Can you work these out from the model? Positions are in its coordinate system, mm. Face numbers are marked on the shaded views. Coordinates: 2 decimals unless noted, no trailing zeros. Order: outer loops, then holes, each group sorted by start corner. A loop starts at its lowest first (then second) coordinate and runs counter-clockwise, first axis right, second up. Notation, with made-up numbers: (72.25, 49) -> (88.25, 49) arc R17 ccw to (88.25, 66) -> close; hole circle Ø4 at (-8, 41). An arc over 180 degrees is marked (long way). Write item = value, one per line.
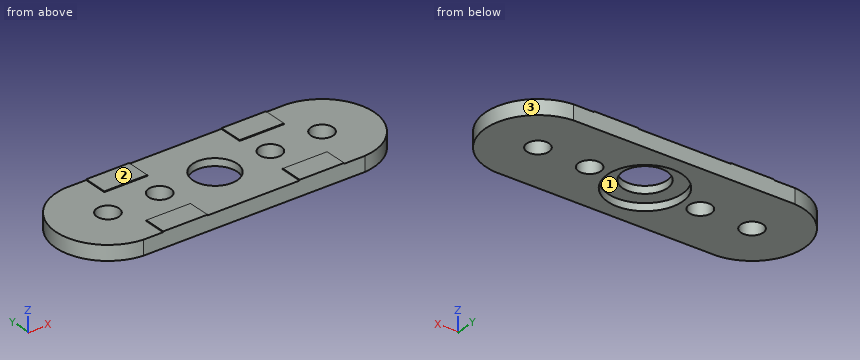
```python
from build123d import *

# Parameters (mm, degrees)
SKETCH1_R           = 3
SKETCH1_R_2         = 1.5
BOSS_EXTRUDE1_DEPTH = 2
SKETCH2_W           = 6.020555891
SKETCH2_H           = 3.042269969
SKETCH2_H_2         = 3.263297615
SKETCH2_W_2         = 6
SKETCH2_W_3         = 5.83801195
BOSS_EXTRUDE2_DEPTH = 0.1
SKETCH3_R           = 5
CUT_EXTRUDE1_DEPTH  = 1


with BuildPart() as part:
    # Sketch1 → Boss-Extrude1 (new body)
    with BuildSketch(Plane.XY):
        with BuildLine():
            Line((-15, -7), (15, -7))
            ThreePointArc((15, -7), (21.517834424, 0), (15, 7))
            Line((15, 7), (-15, 7))
            ThreePointArc((-15, 7), (-21.517834424, 0), (-15, -7))
        make_face()
        Circle(SKETCH1_R, mode=Mode.SUBTRACT)
        with Locations((-14.5, 0)):
            Circle(SKETCH1_R_2, mode=Mode.SUBTRACT)
        with Locations((14.5, 0)):
            Circle(SKETCH1_R_2, mode=Mode.SUBTRACT)
        with Locations((-7.5, 0)):
            Circle(SKETCH1_R_2, mode=Mode.SUBTRACT)
        with Locations((7.5, 0)):
            Circle(SKETCH1_R_2, mode=Mode.SUBTRACT)
    extrude(amount=BOSS_EXTRUDE1_DEPTH)

    # Sketch2 → Boss-Extrude2 (add)
    with BuildSketch(Plane.XY.offset(2)):
        with Locations((9.181574615, -5.478865016)):
            Rectangle(SKETCH2_W, SKETCH2_H)
        with Locations((9.181574615, 5.368351193)):
            Rectangle(SKETCH2_W, SKETCH2_H_2)
        with Locations((-9.322339138, -5.478865016)):
            Rectangle(SKETCH2_W_2, SKETCH2_H)
        with Locations((-9.241345113, 5.368351193)):
            Rectangle(SKETCH2_W_3, SKETCH2_H_2)
    extrude(amount=BOSS_EXTRUDE2_DEPTH)

    # Sketch3 → Cut-Extrude1 (cut)
    with BuildSketch(Plane(origin=(0, 0, 0), x_dir=(-1, 0, 0), z_dir=(0, 0, -1))):
        Circle(SKETCH3_R)
    extrude(amount=-CUT_EXTRUDE1_DEPTH, mode=Mode.SUBTRACT)


solid = part.part
```
Item 1: I want a section at C-C, the plane z = 1.6. Please give me the cut outline in (x, y).
A:
outline = (-15, -7) -> (15, -7) arc R7.02 ccw to (15, 7) -> (-15, 7) arc R7.02 ccw to start; hole circle Ø3 at (-14.5, 0); hole circle Ø3 at (-7.5, 0); hole circle Ø6 at (0, 0); hole circle Ø3 at (7.5, 0); hole circle Ø3 at (14.5, 0)
Item 2: I want a section at B-B, the plane y = 0. Please give me the cut outline in (x, z), plus the area to 3 significant figures.
A:
outline = (-21.52, 0) -> (-16, 0) -> (-16, 2) -> (-21.52, 2) -> close; (-13, 0) -> (-9, 0) -> (-9, 2) -> (-13, 2) -> close; (-6, 0) -> (-5, 0) -> (-5, 1) -> (-3, 1) -> (-3, 2) -> (-6, 2) -> close; (3, 1) -> (5, 1) -> (5, 0) -> (6, 0) -> (6, 2) -> (3, 2) -> close; (9, 0) -> (13, 0) -> (13, 2) -> (9, 2) -> close; (16, 0) -> (21.52, 0) -> (21.52, 2) -> (16, 2) -> close
area = 46.1 mm2
Item 3: I want a section at D-D, the plane y = 2. Please give me the cut outline in (x, z).
A:
outline = (-21.23, 0) -> (-4.58, 0) -> (-4.58, 1) -> (-2.24, 1) -> (-2.24, 2) -> (-21.23, 2) -> close; (2.24, 1) -> (4.58, 1) -> (4.58, 0) -> (21.23, 0) -> (21.23, 2) -> (2.24, 2) -> close
Item 4: I'm going to push a flat-ended pin straight in: P1, Ø1, axis at x = -0.5, y = 4.5, coming from the +Z side. Where does the tip first touch, or does it pass through?
A:
P1 = 2
Item 5: If we mould it in two halves opening along Y, with no side actions, what happens to the marked faces 1, 2 and 3? For each: pulls with the +Y half, pulls with the -Y half, needs draft (parallel to the pull), parting line crosses it, or undercut.
A:
face_1 = undercut
face_2 = needs draft
face_3 = parting line crosses it
Item 6: If I drill on probe 1 along Y at (x, z) = (-4, 0.95); probe 2 along Y at (x, z) = (0, 0.4); probe 3 along Z at (x, y) = (9.5, 0.5), over which ranges is the centre line in solid material (lowest first)?
A:
probe_1 = -7 to -3, 3 to 7
probe_2 = -7 to -5, 5 to 7
probe_3 = 0 to 2
Item 7: I want a section at A-A, the plane x = 14.5. Please give me the cut outline in (y, z), plus the area to 3 significant figures.
A:
outline = (-7, 0) -> (-1.5, 0) -> (-1.5, 2) -> (-7, 2) -> close; (1.5, 0) -> (7, 0) -> (7, 2) -> (1.5, 2) -> close
area = 22.0 mm2
